Geometry check sheet. Reference: the model listing, model coordinates, mm. Round coordinates to 2 decimals unless told otherwise and drop trailing zeros. Order: outer loops, then holes, each group sorted by start corner. A loop starts at its lowest first (then second) coordinate and runs counter-clockwise, first axis right, second up. Notation, with made-up numbers: (80.25, 32) - (121.25, 32) arc R31 cw to (121.25, 58) - close; hole circle Ø8 at (-35, -35). An arc over 180 degrees is marked (long way). Return JSON: item names as keys, results as strings. Group by question number.
Q1. Sectioned sample at A-A, the plane x = 30. Record the cut outline in (y, z), then the cut area to 3 significant figures.
Q2. Sectioned sample at B-B, the plane z = 0.5. Record the cut outline in (x, y), then the cut area to 3 significant figures.
Q3. Material ranges on line 1 along X through (y, z) = (-1.25, 0.55); line 2 along X through (y, z) = (1.75, 0.65); line 3 along Y through (x, z) = (30, 0.2), recorded low to high.
Q4. Sectioned sample at C-C, the plane y = -0.75. Record the cut outline in (x, z), then the cut area to 3 significant figures.
Q5. Draft check along X on faces 1 (the cylindrical face through (-5, 0.1, 0.5)), 2 (the cylindrical face through (37.9, 0.09, 0.49)), 3 (the flat face through (19.7, -5, 0.5)), 4 (the cylindrical face through (45, -0.1, 0.5)). Enter one of: pulls with the +X half, pulls with the -X half, needs draft (parallel to the pull), parting line crosses it, or undercut.
```python
from build123d import *

# Parameters (mm, degrees)
SKETCH_R  = 2.1
PAD_DEPTH = 1


with BuildPart() as part:
    # Sketch → Pad (new body)
    with BuildSketch(Plane.XY):
        with BuildLine():
            ThreePointArc((0, 5), (-5, 0), (0, -5))
            Line((0, -5), (40, -5))
            ThreePointArc((40, -5), (45, 0), (40, 5))
            Line((0, 5), (40, 5))
        make_face()
        Circle(SKETCH_R, mode=Mode.SUBTRACT)
        with Locations((10, 0)):
            Circle(SKETCH_R, mode=Mode.SUBTRACT)
        with Locations((20, 0)):
            Circle(SKETCH_R, mode=Mode.SUBTRACT)
        with Locations((30, 0)):
            Circle(SKETCH_R, mode=Mode.SUBTRACT)
        with Locations((40, 0)):
            Circle(SKETCH_R, mode=Mode.SUBTRACT)
    extrude(amount=PAD_DEPTH)


solid = part.part
```
Reply:
{
 "1": {"outline": "(-5, 0) - (-2.1, 0) - (-2.1, 1) - (-5, 1) - close; (2.1, 0) - (5, 0) - (5, 1) - (2.1, 1) - close", "area": "5.80 mm^2"},
 "2": {"outline": "(0, -5) - (40, -5) arc R5 ccw to (40, 5) - (0, 5) arc R5 ccw to start; hole circle Ø4.2 at (0, 0); hole circle Ø4.2 at (10, 0); hole circle Ø4.2 at (20, 0); hole circle Ø4.2 at (30, 0); hole circle Ø4.2 at (40, 0)", "area": "409 mm^2"},
 "3": {"line 1": "-4.84 to -1.69, 1.69 to 8.31, 11.69 to 18.31, 21.69 to 28.31, 31.69 to 38.31, 41.69 to 44.84", "line 2": "-4.68 to -1.16, 1.16 to 8.84, 11.16 to 18.84, 21.16 to 28.84, 31.16 to 38.84, 41.16 to 44.68", "line 3": "-5 to -2.1, 2.1 to 5"},
 "4": {"outline": "(-4.94, 0) - (-1.96, 0) - (-1.96, 1) - (-4.94, 1) - close; (1.96, 0) - (8.04, 0) - (8.04, 1) - (1.96, 1) - close; (11.96, 0) - (18.04, 0) - (18.04, 1) - (11.96, 1) - close; (21.96, 0) - (28.04, 0) - (28.04, 1) - (21.96, 1) - close; (31.96, 0) - (38.04, 0) - (38.04, 1) - (31.96, 1) - close; (41.96, 0) - (44.94, 0) - (44.94, 1) - (41.96, 1) - close", "area": "30.3 mm^2"},
 "5": {"face 1": "pulls with the -X half", "face 2": "undercut", "face 3": "needs draft", "face 4": "pulls with the +X half"}
}
